Build history of the part. All positions in model axes, mm. A direction names the side the tool comes from. Give positions to 0.01 mm unless a question says otherwise; leave off trailing zeros. Write each loop counter-clockwise with the first axis right and the second up, starting at its lowest first coordinate (ties: lowest second). Pieces come first, ordered by that corner, then holes.
from build123d import *

# Parameters (mm, degrees)
F2_R     = 88.9
F4_DEPTH = 127


# Not quite as in the source:
# - the program builds the solid bodies; features that only make, move or delete a surface that nothing else refers to are left out


with BuildPart() as f1:
    # F0 (on Front) → F1 (revolve)
    with BuildSketch(Plane.XZ):
        Polygon((-17.8278337446, 25.4), (0, 25.4), (55.6368945653, 25.4), (55.6368945653, 50.8), (47.4307299643, 50.8), (47.4307299643, 127), (-17.8278337446, 127), (-17.8278337446, 121.92), (-26.8155404944, 121.92), (-26.8155404944, 30.48), (-17.8278337446, 30.48), align=None)
    revolve(axis=Axis((17.3414491085, 0, 0), (1, 0, 0)))

    # F2 (on Right) → F4 (join)
    with BuildSketch(Plane.YZ):
        Circle(F2_R)
    extrude(amount=F4_DEPTH)


solid = f1.part
(1) Saw through at C-C, the plane x = 11. List the corners of the cut face in (y, z).
(2) Saw through at B-B, the plane z = 73.5. List the corners of the cut face in (x, y).
(3) Mould opens along Z. For faces 1 (the face through (-26.816, 25, 25)), 2 (the face through (0, 0, 0)), 3 (the face through (86.658, 84.795, 26.703)) say: +Z half, -Z half, draft (parallel to the pull), parting line (faces both ways), or undercut.
(4) Saw through at A-A, the plane y = 0. List the corners of the cut face in (x, z).
(5) Probe line 1 (Z direction, x = -7, y = 0); line 2 (Y direction, x = -22.75, z = 0). List the from-to ranges inside material, lowest first.
(6) Drop flat-ended pins along their axis: pin 1 (2 mm diameter, centred on x = 96.5, y = 41.5, fed in from +Z); pin 2 (2 mm diameter, centred on x = 80, z = -9, fed in from +Y); pin 3 (12 mm diameter, centred on x = 80.5, z = 29.5, fed in from +Y). Give the stop position or say it passes through.
(7) 3-axis set-ups, long thin cutter, end or side, ignore diameter. For faces 4 (the face through (-17.828, -25, -7)), 5 (the face through (14.34, 123.98, -27.53)), 6 (the face through (47.431, 26, 86)): which of +Z, -Z, +X, -X, +Y, -Y reach the whole face in a straight line?
Computed values:
1. outline: circle Ø254 at (0, 0)
2. outline: (-26.82, -97.27) - (-17.83, -97.27) - (-17.83, -103.57) - (47.43, -103.57) - (47.43, -50.01) - (127, -50.01) - (127, 50.01) - (47.43, 50.01) - (47.43, 103.57) - (-17.83, 103.57) - (-17.83, 97.27) - (-26.82, 97.27) - close
3. face 1: draft
3. face 2: undercut
3. face 3: parting line
4. outline: (-26.82, -121.92) - (-17.83, -121.92) - (-17.83, -127) - (47.43, -127) - (47.43, -88.9) - (127, -88.9) - (127, 88.9) - (47.43, 88.9) - (47.43, 127) - (-17.83, 127) - (-17.83, 121.92) - (-26.82, 121.92) - (-26.82, 30.48) - (-17.83, 30.48) - (-17.83, 25.4) - (0, 25.4) - (0, -25.4) - (-17.83, -25.4) - (-17.83, -30.48) - (-26.82, -30.48) - close
5. line 1: z = -127 to -25.4, 25.4 to 127
5. line 2: y = -121.92 to -30.48, 30.48 to 121.92
6. pin 1: stops at z = 79.14
6. pin 2: stops at y = 88.54
6. pin 3: stops at y = 85.74
7. face 4: -X
7. face 5: +X, -X
7. face 6: +X
